The model under review builds one solid part; all positions refer to its coordinate system, in mm. A direction names the side the tool comes from. Round coordinates to 2 decimals unless told otherwise and drop trailing zeros. Order: outer loops, then holes, each group sorted by start corner. A loop starts at its lowest first (then second) coordinate and runs counter-clockwise, first axis right, second up. Notation, with made-up numbers: M 31,25.25 L 50,25.25 A17 ccw 50,30.25 Z; hole C 76,62.25 d3. An arc over 180 degrees is marked long. Use a Markdown table: item, result. Add a question column.
1. Consider section B-B on y = 98. State the section outline as (x, z) points.
2. Consider section C-C on y = 143. State the section outline as (x, z) points, then the cut area to 3 significant figures.
3. To check wall thickness, follow probe 1 along Y at (x, z) = (12.7, 0.6); probe 2 along X at (y, z) = (193.5, 0.9); probe 3 along Y at (x, z) = (79, 1) (3 decimals). State the ranges of each line that lie inside material, in increasing order.
4. Consider section D-D on x = 170.5. State the section outline as (y, z) points, then the cut area to 3 significant figures.
5. The part is to be moulded in two halves that separate along X. For faces 4 (the flat face through (113, 80, 1.27)), 5 (the cylindrical face through (178.5, 1.26, 0.63)), 6 (the cylindrical face through (224.78, 199.58, 0.64)), say which applies: +X half, -X half, draft (parallel to the pull), parting line (faces both ways), or undercut.
6. Insertion check: P1, Ø0.6, axis at x = 128, z = 0.5, coming from the +Y side; P2, Ø5.5, axis at x = 12.7, y = 190.5, coming from the +Z side. Each pin has a flat end and moves straight along its axis. Give the tip position at first contact, or say it passes through.
7. For faces 1 (the cylindrical face through (132.791, 55.823, 0.626)), 2 (the flat face through (68.883, 39.459, 0.644)), 3 (the flat face through (155.317, 174.294, 0.644)), list the 3-axis set-ups (+Z, -Z, +X, -X, +Y, -Y) from which the entire face can be reached by the end or side of a thin tool; tool diameter is ignored.
8. Consider section A-A on x = 206.5. State the section outline as (y, z) points, then the cut area to 3 significant figures.
from build123d import *

# Parameters (mm, degrees)
F0_W     = 228.6
F0_H     = 203.2
F1_DEPTH = 1.27
F2_R     = 3.5687
F3_DEPTH = 1.271
F5_DEPTH = 25.4
F6_R     = 12.7
F8_DEPTH = 25.4


with BuildPart() as f1:
    # F0 (on Top) → F1 (new body)
    with BuildSketch(Plane.XY):
        with Locations((114.3, 101.6)):
            Rectangle(F0_W, F0_H)
    extrude(amount=F1_DEPTH)

    # F2 (on face) → F3 (cut, through all)
    with BuildSketch(Plane.XY.offset(1.27)):
        with BuildLine():
            Line((38.1, 128.0287), (12.7, 128.0287))
            ThreePointArc((12.7, 128.0287), (9.1313, 124.46), (12.7, 120.8913))
            Line((12.7, 120.8913), (38.1, 120.8913))
            ThreePointArc((38.1, 120.8913), (41.6687, 124.46), (38.1, 128.0287))
        make_face()
        with BuildLine():
            Line((215.9, 128.0287), (190.5, 128.0287))
            ThreePointArc((190.5, 128.0287), (186.9313, 124.46), (190.5, 120.8913))
            Line((190.5, 120.8913), (215.9, 120.8913))
            ThreePointArc((215.9, 120.8913), (219.4687, 124.46), (215.9, 128.0287))
        make_face()
        with BuildLine():
            Line((38.1, 82.3087), (12.7, 82.3087))
            ThreePointArc((12.7, 82.3087), (9.1313, 78.74), (12.7, 75.1713))
            Line((12.7, 75.1713), (38.1, 75.1713))
            ThreePointArc((38.1, 75.1713), (41.6687, 78.74), (38.1, 82.3087))
        make_face()
        with BuildLine():
            ThreePointArc((190.5, 82.3087), (186.9313, 78.74), (190.5, 75.1713))
            Line((190.5, 75.1713), (215.9, 75.1713))
            ThreePointArc((215.9, 75.1713), (219.4687, 78.74), (215.9, 82.3087))
            Line((215.9, 82.3087), (190.5, 82.3087))
        make_face()
        with Locations((12.7, 190.5)):
            Circle(F2_R)
        with Locations((215.9, 190.5)):
            Circle(F2_R)
        with Locations((12.7, 12.7)):
            Circle(F2_R)
        with Locations((215.9, 12.7)):
            Circle(F2_R)
    extrude(amount=-F3_DEPTH, mode=Mode.SUBTRACT)

    # F4 (on face) → F5 (cut)
    with BuildSketch(Plane.XY.offset(1.27)):
        Polygon((50.8, 203.2), (101.6, 146.05), (133.35, 146.05), (177.8, 203.2), align=None)
        Polygon((133.35, 57.15), (101.6, 57.15), (50.8, 0), (177.8, 0), align=None)
    extrude(amount=-F5_DEPTH, mode=Mode.SUBTRACT)

    # F6
    f6_edges = [f1.edges().sort_by_distance(p)[0] for p in [
        (50.8, 0, 0.635),
        (101.6, 57.15, 0.635),
        (0, 0, 0.635),
        (133.35, 57.15, 0.635),
        (177.8, 0, 0.635),
        (228.6, 0, 0.635),
        (228.6, 203.2, 0.635),
        (177.8, 203.2, 0.635),
        (133.35, 146.05, 0.635),
        (101.6, 146.05, 0.635),
        (50.8, 203.2, 0.635),
        (0, 203.2, 0.635),
    ]]
    fillet(f6_edges, radius=F6_R)

    # F7 (on face) → F8 (cut)
    with BuildSketch(Plane.XY.offset(1.27)):
        with BuildLine():
            Line((90.2719138145, 139.6780655649), (48.0848100488, 187.1385573013))
            ThreePointArc((48.0848100488, 187.1385573013), (34.6376707235, 187.9295654969), (33.8466625279, 174.4824261716))
            Line((33.8466625279, 174.4824261716), (76.0337662936, 127.0219344351))
            ThreePointArc((76.0337662936, 127.0219344351), (89.4809056189, 126.2309262395), (90.2719138145, 139.6780655649))
        make_face()
        with BuildLine():
            ThreePointArc((144.1698608703, 139.6780655649), (144.9608690659, 126.2309262395), (158.4080083912, 127.0219344351))
            Line((158.4080083912, 127.0219344351), (200.5951121569, 174.4824261716))
            ThreePointArc((200.5951121569, 174.4824261716), (199.8041039613, 187.9295654969), (186.356964636, 187.1385573013))
            Line((186.356964636, 187.1385573013), (144.1698608703, 139.6780655649))
        make_face()
        with BuildLine():
            ThreePointArc((90.2719138145, 63.5219344351), (89.4809056189, 76.9690737605), (76.0337662936, 76.1780655649))
            Line((76.0337662936, 76.1780655649), (33.8466625279, 28.7175738284))
            ThreePointArc((33.8466625279, 28.7175738284), (34.6376707235, 15.2704345031), (48.0848100488, 16.0614426987))
            Line((48.0848100488, 16.0614426987), (90.2719138145, 63.5219344351))
        make_face()
        with BuildLine():
            Line((200.5951121569, 28.7175738284), (158.4080083912, 76.1780655649))
            ThreePointArc((158.4080083912, 76.1780655649), (144.9608690659, 76.9690737605), (144.1698608703, 63.5219344351))
            Line((144.1698608703, 63.5219344351), (186.356964636, 16.0614426987))
            ThreePointArc((186.356964636, 16.0614426987), (199.8041039613, 15.2704345031), (200.5951121569, 28.7175738284))
        make_face()
        with BuildLine():
            ThreePointArc((66.4208873424, 114.3), (53.7208873424, 101.6), (66.4208873424, 88.9))
            Line((66.4208873424, 88.9), (117.2208873424, 88.9))
            Line((117.2208873424, 88.9), (168.0208873424, 88.9))
            ThreePointArc((168.0208873424, 88.9), (180.7208873424, 101.6), (168.0208873424, 114.3))
            Line((168.0208873424, 114.3), (117.2208873424, 114.3))
            Line((117.2208873424, 114.3), (66.4208873424, 114.3))
        make_face()
    extrude(amount=-F8_DEPTH, mode=Mode.SUBTRACT)


solid = f1.part
Answer block:
| question | item | result |
|---|---|---|
| 1 | outline | M 0,0 L 54.24,0 L 54.24,1.27 L 0,1.27 Z; M 180.2,0 L 228.6,0 L 228.6,1.27 L 180.2,1.27 Z |
| 2 | outline | M 0,0 L 61.83,0 L 61.83,1.27 L 0,1.27 Z; M 87.32,0 L 147.12,0 L 147.12,1.27 L 87.32,1.27 Z; M 172.61,0 L 228.6,0 L 228.6,1.27 L 172.61,1.27 Z |
| 2 | area | 226 mm^2 |
| 3 | probe 1 | 0 to 9.13, 16.27 to 75.17, 82.31 to 120.89, 128.03 to 186.93, 194.07 to 203.2 |
| 3 | probe 2 | 0.36 to 10.77, 14.63 to 59.42, 170.26 to 213.97, 217.83 to 228.24 |
| 3 | probe 3 | 31.725 to 50.841, 78.422 to 88.9, 114.3 to 124.778, 152.359 to 171.475 |
| 4 | outline | M 9.39,0 L 33.9,0 L 33.9,1.27 L 9.39,1.27 Z; M 62.57,0 L 89.14,0 L 89.14,1.27 L 62.57,1.27 Z; M 114.06,0 L 140.63,0 L 140.63,1.27 L 114.06,1.27 Z; M 169.3,0 L 193.81,0 L 193.81,1.27 L 169.3,1.27 Z |
| 4 | area | 130 mm^2 |
| 5 | face 4 | draft |
| 5 | face 5 | undercut |
| 5 | face 6 | +X half |
| 6 | P1 | y = 146.1 |
| 6 | P2 | through |
| 7 | face 1 | +Z, -Z, -Y |
| 7 | face 2 | +Z, -Z |
| 7 | face 3 | +Z, -Z, +Y |
| 8 | outline | M 0,0 L 75.17,0 L 75.17,1.27 L 0,1.27 Z; M 82.31,0 L 120.89,0 L 120.89,1.27 L 82.31,1.27 Z; M 128.03,0 L 203.2,0 L 203.2,1.27 L 128.03,1.27 Z |
| 8 | area | 240 mm^2 |
